```python
from build123d import *

# Parameters (mm, degrees)
SKETCH_W        = 84
SKETCH_H        = 84
PAD_DEPTH       = 7
SKETCH006_W     = 13.4
SKETCH006_H     = 13.4
SKETCH006_R     = 3.25
POCKET_DEPTH    = 5
SKETCH004_R     = 2.4
PAD001_DEPTH    = 3
SKETCH011_W     = 84
SKETCH011_H     = 84
SKETCH011_W_2   = 17.8
SKETCH011_H_2   = 17.8
PAD002_DEPTH    = 3
SKETCH005_W     = 13
SKETCH005_H     = 44
POCKET001_DEPTH = 10.001
SKETCH012_W     = 48.1
SKETCH012_H     = 5
POCKET002_DEPTH = 84.001
SKETCH013_W     = 48.1
SKETCH013_H     = 5
POCKET003_DEPTH = 84.001


with BuildPart() as part:
    # Sketch → Pad (new body)
    with BuildSketch(Plane.XY):
        Rectangle(SKETCH_W, SKETCH_H)
    extrude(amount=PAD_DEPTH)

    # Sketch006 → Pocket (cut)
    with BuildSketch(Plane(origin=(0, 0, 0), x_dir=(1, 0, 0), z_dir=(0, 0, -1))):
        with Locations((-31.95, 31.95)):
            Rectangle(SKETCH006_W, SKETCH006_H)
        with Locations((-31.95, 31.95)):
            Circle(SKETCH006_R, mode=Mode.SUBTRACT)
        with Locations((31.95, 31.95)):
            Rectangle(SKETCH006_W, SKETCH006_H)
        with Locations((31.95, 31.95)):
            Circle(SKETCH006_R, mode=Mode.SUBTRACT)
        with Locations((-31.95, -31.95)):
            Rectangle(SKETCH006_W, SKETCH006_H)
        with Locations((-31.95, -31.95)):
            Circle(SKETCH006_R, mode=Mode.SUBTRACT)
        with Locations((31.95, -31.95)):
            Rectangle(SKETCH006_W, SKETCH006_H)
        with Locations((31.95, -31.95)):
            Circle(SKETCH006_R, mode=Mode.SUBTRACT)
        Polygon((-42, -24.05), (-42, -42), (-24.05, -42), (-24.05, -39.85), (-39.85, -39.85), (-39.85, -24.05), align=None)
        Polygon((24.05, -42), (42, -42), (42, -24.05), (39.85, -24.05), (39.85, -39.85), (24.05, -39.85), align=None)
        Polygon((42, 24.05), (42, 42), (24.05, 42), (24.05, 39.85), (39.85, 39.85), (39.85, 24.05), align=None)
        Polygon((-42, 24.05), (-42, 42), (-24.05, 42), (-24.05, 39.85), (-39.85, 39.85), (-39.85, 24.05), align=None)
    extrude(amount=-POCKET_DEPTH, mode=Mode.SUBTRACT)

    # Sketch004 → Pad001 (new body)
    with BuildSketch(Plane.XY.offset(7)):
        with Locations((-35.95, -35.95)):
            Circle(SKETCH004_R)
        with Locations((35.95, 35.95)):
            Circle(SKETCH004_R)
        with Locations((35.95, -35.95)):
            Circle(SKETCH004_R)
        with Locations((-35.95, 35.95)):
            Circle(SKETCH004_R)
        with Locations((-27.95, 35.95)):
            Circle(SKETCH004_R)
        with Locations((-27.95, 27.95)):
            Circle(SKETCH004_R)
        with Locations((27.95, 27.95)):
            Circle(SKETCH004_R)
        with Locations((27.95, 35.95)):
            Circle(SKETCH004_R)
        with Locations((-35.95, 27.95)):
            Circle(SKETCH004_R)
        with Locations((35.95, 27.95)):
            Circle(SKETCH004_R)
        with Locations((27.95, -27.95)):
            Circle(SKETCH004_R)
        with Locations((27.95, -35.95)):
            Circle(SKETCH004_R)
        with Locations((35.95, -27.95)):
            Circle(SKETCH004_R)
        with Locations((-27.95, -27.95)):
            Circle(SKETCH004_R)
        with Locations((-27.95, -35.95)):
            Circle(SKETCH004_R)
        with Locations((-35.95, -27.95)):
            Circle(SKETCH004_R)
    extrude(amount=PAD001_DEPTH)

    # Sketch011 → Pad002 (new body)
    with BuildSketch(Plane.XY.offset(7)):
        Rectangle(SKETCH011_W, SKETCH011_H)
        with Locations((-32.1, 32.1)):
            Rectangle(SKETCH011_W_2, SKETCH011_H_2, mode=Mode.SUBTRACT)
        with Locations((-32.1, -32.1)):
            Rectangle(SKETCH011_W_2, SKETCH011_H_2, mode=Mode.SUBTRACT)
        with Locations((32.1, 32.1)):
            Rectangle(SKETCH011_W_2, SKETCH011_H_2, mode=Mode.SUBTRACT)
        with Locations((32.1, -32.1)):
            Rectangle(SKETCH011_W_2, SKETCH011_H_2, mode=Mode.SUBTRACT)
    extrude(amount=PAD002_DEPTH)

    # Sketch005 → Pocket001 (cut, through all)
    with BuildSketch(Plane.XY.offset(10)):
        with Locations((-31.5, 0)):
            Rectangle(SKETCH005_W, SKETCH005_H)
    extrude(amount=-POCKET001_DEPTH, mode=Mode.SUBTRACT)

    # Sketch012 → Pocket002 (cut, through all)
    with BuildSketch(Plane.XZ.offset(42)):
        with Locations((0, 2.5)):
            Rectangle(SKETCH012_W, SKETCH012_H)
    extrude(amount=-POCKET002_DEPTH, mode=Mode.SUBTRACT)

    # Sketch013 → Pocket003 (cut, through all)
    with BuildSketch(Plane.YZ.offset(42)):
        with Locations((0, 2.5)):
            Rectangle(SKETCH013_W, SKETCH013_H)
    extrude(amount=-POCKET003_DEPTH, mode=Mode.SUBTRACT)


solid = part.part
```
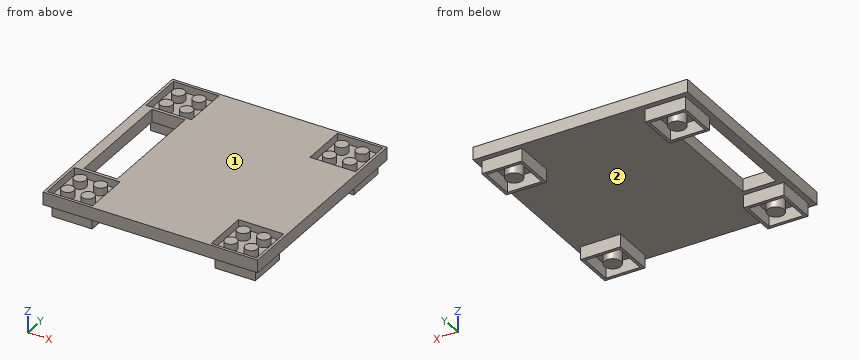
Work out the finished part from the listing and answer in its coordinate system (mm). Face numbers are marked on the shaded views. Give positions to 0.01 mm unless a question says otherwise; leave off trailing zeros. Loops run counter-clockwise (first coordinate to the right, second up) from the corner with the lowest first, then second, coordinate; pieces in that order, holes last. Notation, with made-up numbers: (22.25, 42.5) -> (52.25, 42.5) arc R17 ccw to (52.25, 54.5) -> close; hole circle Ø5 at (27.5, 51). An arc over 180 degrees is marked (long way). Put each result on its own line as item: value. Start each with the question number.
Item 1: Each of these flat-tipped pins is pushed along its axis until it touches: P1, Ø4, axis at x = 32, z = 2.5, coming from the +Y side; P2, Ø3, axis at x = -9, z = 2, coming from the -Y side; P3, Ø2.5, axis at x = -28, z = 2, coming from the -Y side; P4, Ø1.5, axis at y = 33, z = 2, coming from the -X side. Where does it stop, or does it pass through?
Item 2: The part is cut by section A-A (y = -14). Give the vertices of the cut face in (x, z).
Item 3: Find the intervals of material crossed by L1, parallel to Y at x = -28, z = 3.5; L2, parallel to X at y = -1, z = 7.5, in increasing order. Write a range as [from, to].
Item 4: The part is cut by section B-B (x = -13.5). Give the vertices of the cut face in (y, z).
Item 5: The mould has two halves that part along X. Classify the marked faces 1 and 2: released by +X, released by -X, zero draft, split by the parting line, or undercut.
Answers below:
1. P1: y = 39.85
1. P2: through
1. P3: y = -39.85
1. P4: x = -39.85
2. outline: (-42, 5) -> (-38, 5) -> (-38, 10) -> (-42, 10) -> close; (-25, 5) -> (42, 5) -> (42, 10) -> (-25, 10) -> close
3. L1: [-39.85, -38.65], [-25.25, -24.05], [24.05, 25.25], [38.65, 39.85]
3. L2: [-42, -38], [-25, 42]
4. outline: (-42, 5) -> (42, 5) -> (42, 10) -> (-42, 10) -> close
5. face 1: zero draft
5. face 2: undercut
